Autodesk Fusion 360 part; units mm, degrees
sketch "Sketch1" plane through (0, 0, 0) normal (0, 1, 0) x (1, 0, 0)
  line L0 (0, 0) -> (4, 0)
  arc A0 (5, -1) -> (4, 0) centre (4, -1) ccw
  line L1 (5, -1) -> (5, -13)
  line L2 (0, 0) -> (0, -30)
  line L3 (0, -30) -> (2, -30)
  spline S0 degree 2 poles (5, -13) (4.7977, -14.1987) (4, -15) knots 0 0 0 0.22987 0.22987 0.22987 weights 1 3 1
  arc A1 (2, -30) -> (2, -28.5) centre (1.7031, -29.25) ccw
  line L4 (2, -28.5) -> (2, -26.5)
  spline S1 degree 2 poles (4, -15) (2.6442, -16.1662) (2, -26.5) knots 0 0 0 1.18535 1.18535 1.18535 weights 1 3 1
  dimension "d1" = 4
  dimension "d2" = 12
  dimension "d3" = 30
  dimension "d9" = 2
  dimension "d11" = 2
revolve "Revolve1" add sketch "Sketch1" angle 360 about axis through (0, 0, 0) along (0, 0, 1)
The listing builds one solid part. Answer for the finished solid, in the listing's coordinates (mm). Round coordinates to 2 decimals unless told otherwise and drop trailing zeros. Loops run counter-clockwise (first coordinate to the right, second up) from the corner with the lowest first, then second, coordinate; pieces in that order, holes last.
Q1. Given pin 1 Ø6 at (x, z) = (1, 16) entering from -Y; pin 2 Ø5 at (x, y) = (0, 3) entering from +Z, each flat-ended and moving along its own axis, determine where each tip first touches the part or whether it passes through.
Q2. Section A-A, the plane z = 8.5 is taken. Determine the outline of the cut face in (x, y), then the cut area to 3 significant figures.
Q3. For a pull along Z with two mould halves and no side action, classify faces 1 (the face through (-1.08, -4.88, 7.08)), 2 (the face through (0, 0, 0)), 3 (the face through (0, 0, 30)), 4 (the face through (0, 2, 27)) as released by +Z, released by -Z, zero draft, split by the parting line, or undercut.
Q4. Find the intervals of material crossed by line 1 (Y direction, x = -3.5, z = 6.5); line 2 (X direction, y = -1.5, z = 11); line 3 (Y direction, x = 3.75, z = 6.5), in increasing order.
Completed:
1. pin 1: stops at y = -4.98
1. pin 2: stops at z = 30
2. outline: circle Ø10 at (0, 0)
2. area: 78.5 mm2
3. face 1: zero draft
3. face 2: released by -Z
3. face 3: released by +Z
3. face 4: undercut
4. line 1: y = -3.57 to 3.57
4. line 2: x = -4.77 to 4.77
4. line 3: y = -3.31 to 3.31
